Answer from the drawing. Dimensions are ordinates in mm from the lowest x, y and z of the part. A direction names the side the tool comes from. Round coordinates to 2 decimals unless told otherwise and drop trailing zeros. Loops run counter-clockwise (first coordinate to the right, second up) from the corner with the lowest first, then second, coordinate; pieces in that order, holes last. Notation, with made-up numbers: (-16, 14) - (0, 14) arc R18 ccw to (0, 39) - close; hole circle Ø4 at (-28.75, 63.25). An arc over 180 degrees is marked (long way). Answer as CSV lines item,"result". Start each with the question number.
Q1. Section C-C on z = 10 is taken. Write down the section's boundary in (x, y), then the cut area to 3 significant figures.
Q2. Section A-A on y = 14 is taken. Write down the section's boundary in (x, z).
Q3. The mould has two halves that part along X. Classify the marked faces 1, 2 and 3: +X half, -X half, draft (parallel to the pull), parting line (faces both ways), or undercut.
Q4. Section D-D on y = 10 is taken. Write down the section's boundary in (x, z), then the cut area to 3 significant figures.
Q5. Straight lines are drawn through the part: L1, parallel to Y at x = 2.5, z = 10; L2, parallel to X at y = 32.6, z = 10; L3, parallel to X at y = 28.5, z = 8. For each, find the intervals that lie inside material, in ascending order. Write a range as [from, to].
Q6. For the marked faces 4, 5, 6 and 7, determine the directions among +Z, -Z, +X, -X, +Y, -Y from which every point of the face is accessible in a straight line to the end or side of a thin tool.
Q7. Each of these flat-tipped pins is pushed along its axis until it touches: pin 1 Ø7.5 at (x, y) = (39.5, 18.5) entering from -Z; pin 2 Ø3 at (x, z) = (31.5, 14) entering from -Y; pin 3 Ø4 at (y, z) = (13, 4) entering from +X; pin 4 Ø7.5 at (x, y) = (42, 19.5) entering from +Z. Where does it stop, or does it pass through?
Q8. Section B-B on x = 22 is taken. Write down the section's boundary in (y, z).
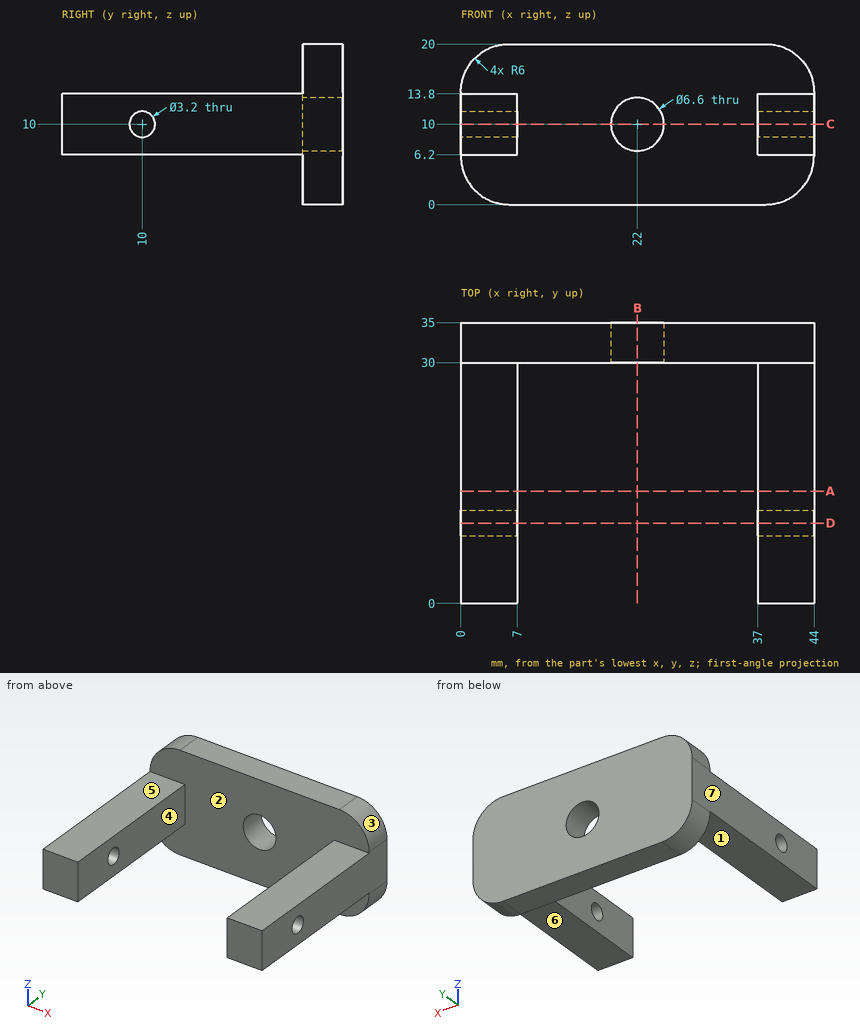
Findings:
1,outline,"(0, 0) - (7, 0) - (7, 8.4) - (0, 8.4) - close; (0, 11.6) - (7, 11.6) - (7, 30) - (18.7, 30) - (18.7, 35) - (0, 35) - close; (25.3, 30) - (37, 30) - (37, 11.6) - (44, 11.6) - (44, 35) - (25.3, 35) - close; (37, 0) - (44, 0) - (44, 8.4) - (37, 8.4) - close"
1,area,"562 mm^2"
2,outline,"(0, 6.2) - (7, 6.2) - (7, 13.8) - (0, 13.8) - close; (37, 6.2) - (44, 6.2) - (44, 13.8) - (37, 13.8) - close"
3,face 1,"draft"
3,face 2,"undercut"
3,face 3,"+X half"
4,outline,"(0, 6.2) - (7, 6.2) - (7, 8.4) - (0, 8.4) - close; (0, 11.6) - (7, 11.6) - (7, 13.8) - (0, 13.8) - close; (37, 6.2) - (44, 6.2) - (44, 8.4) - (37, 8.4) - close; (37, 11.6) - (44, 11.6) - (44, 13.8) - (37, 13.8) - close"
4,area,"61.6 mm^2"
5,L1,"y = [0, 8.4], [11.6, 35]"
5,L2,"x = [0, 18.7], [25.3, 44]"
5,L3,"x = [0, 7], [37, 44]"
6,face 4,"+Z, -Z, -Y"
6,face 5,"+Z, +X, -X, -Y"
6,face 6,"-Z, +X, -X, -Y"
6,face 7,"+Z, -Z, -X, +Y, -Y"
7,pin 1,"stops at z = 6.2"
7,pin 2,"stops at y = 30"
7,pin 3,"passes through"
7,pin 4,"stops at z = 13.8"
8,outline,"(30, 0) - (35, 0) - (35, 6.7) - (30, 6.7) - close; (30, 13.3) - (35, 13.3) - (35, 20) - (30, 20) - close"
